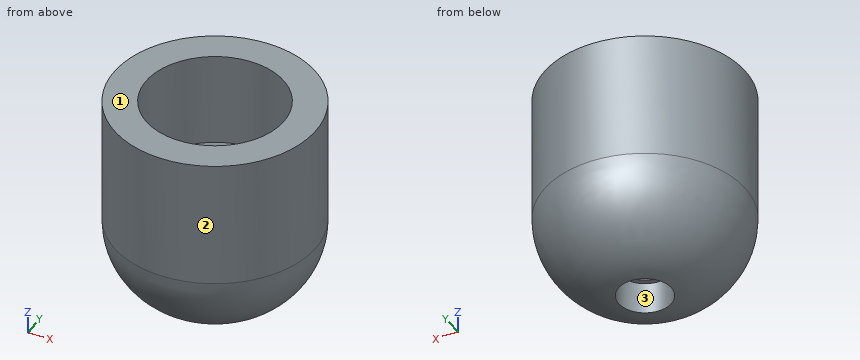
from build123d import *

# Parameters (mm, degrees)
F0_R     = 6.5
F0_R_2   = 2.5
F1_DEPTH = 3
F0_R_3   = 9.5
F2_DEPTH = 20


# Not quite as in the source:
# - a fillet or chamfer that OpenCascade refuses, or shapes differently, is made with other operations: its cross-section is extruded or revolved along the edge and cut away or added


with BuildPart() as f1:
    # F0 (on Top) → F1 (new body)
    with BuildSketch(Plane.XY):
        Circle(F0_R)
        Circle(F0_R_2, mode=Mode.SUBTRACT)
    extrude(amount=F1_DEPTH)

    # F0 (on Top) → F2 (join)
    with BuildSketch(Plane.XY):
        Circle(F0_R_3)
        Circle(F0_R, mode=Mode.SUBTRACT)
    extrude(amount=F2_DEPTH)

    # F3: fillet of radius 8 on 1 edges, made by hand

    # F3_s1 → F3_t2 (revolve, cut)
    with BuildSketch(Plane.XZ):
        with BuildLine():
            ThreePointArc((2.5, 0), (7.5, 2.6457513111), (9.5, 7.9372539332))
            Line((9.5, 7.9372539332), (9.5, 0))
            Line((9.5, 0), (2.5, 0))
        make_face()
    revolve(axis=Axis((0, 0, 0), (0, 0, 1)), mode=Mode.SUBTRACT)

    # F4 (on Right) → F5 (revolve)
    with BuildSketch(Plane.YZ):
        Polygon((7.5, 13), (2, 3), (7.5, 3), align=None)
    revolve(axis=Axis((0, 0, 1.5), (0, 0, 1)))


solid = f1.part
Input: part model. Units: mm. Frame: model coordinates. Face numbers are marked on the shaded views. Give positions to 0.01 mm unless a question says otherwise; leave off trailing zeros. Loops run counter-clockwise (first coordinate to the right, second up) from the corner with the lowest first, then second, coordinate; pieces in that order, holes last. Notation, with made-up numbers: M -10,45 L 44,45 A24 ccw 44,83 Z; hole C 55,41.5 d9. An arc over 180 degrees is marked long. Use CSV: the item, a comma, the result in double quotes.
(1) Material intervals for L1, parallel to Y at x = 0, z = 16; L2, parallel to X at y = 2.5, z = 10.5; L3, parallel to Y at x = 2.5, z = 16.75, sorted ascending. Write a range as [from, to].
Outcome:
L1,"y = [-9.5, -6.5], [6.5, 9.5]"
L2,"x = [-9.17, -5.59], [5.59, 9.17]"
L3,"y = [-9.17, -6], [6, 9.17]"
(2) Section A-A, the plane z = 18.5. Return loops of the section in (x, y).
Outcome:
outline,"C 0,0 d19; hole C 0,0 d13"
(3) Pin query (flat end, axial travel): P1, Ø3, axis at y = 5.5, z = 14, coming from the -X side; P2, Ø6, axis at y = -6, z = 5, coming from the -X side; P3, Ø6, axis at x = 0, y = 0, coming from the +Z side; P4, Ø6, axis at x = -2, z = 10, coming from the -Y side. Return the tip coordinate at first contact, or that it passes through.
Outcome:
P1,"stops at x = -8.62"
P2,"stops at x = -8.73"
P3,"stops at z = 4.82"
P4,"stops at y = -9.5"
(4) Pull-direction query (Y, two-part tool) for the marked faces 1, 2 and 3; classes: pulls with the +Y half, pulls with the -Y half, needs draft (parallel to the pull), parting line crosses it, or undercut.
Outcome:
face 1,"needs draft"
face 2,"parting line crosses it"
face 3,"undercut"
